Geometry check sheet. Reference: drawing and pictorial views, mm from the part's lowest x, y, z. Round coordinates to 2 decimals unless told otherwise and drop trailing zeros. Order: outer loops, then holes, each group sorted by start corner. A loop starts at its lowest first (then second) coordinate and runs counter-clockwise, first axis right, second up.
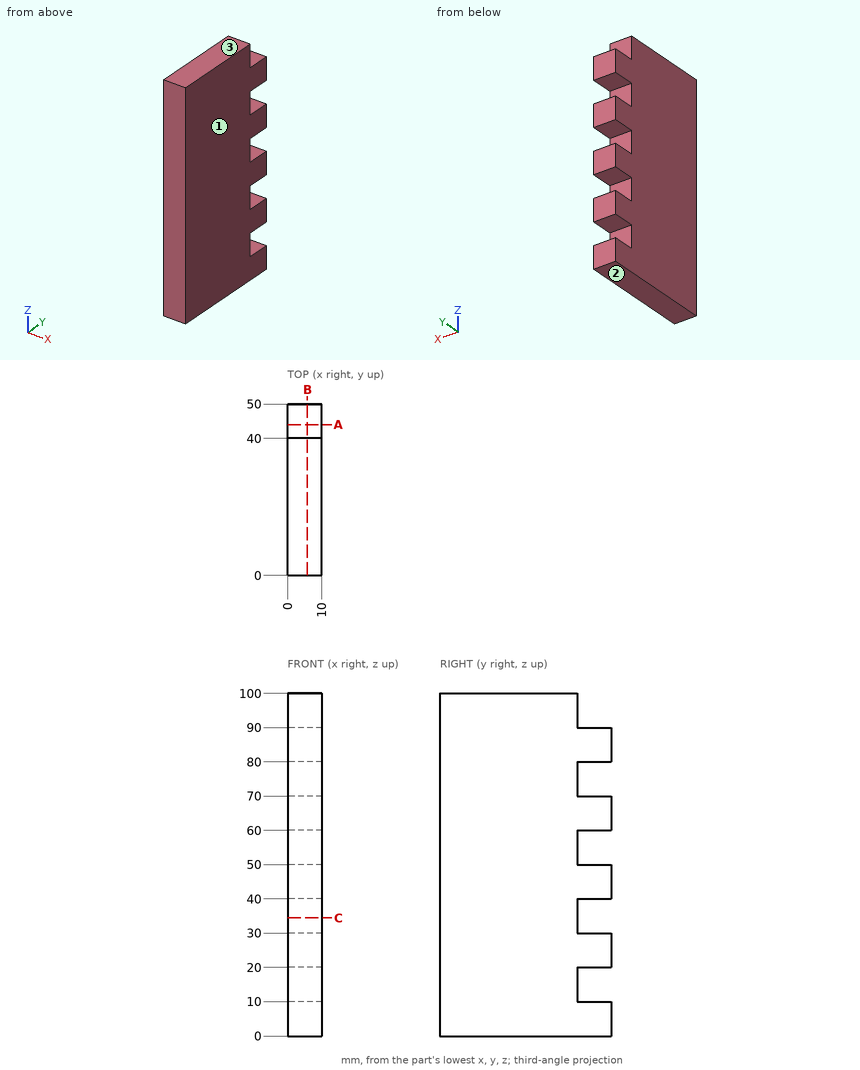
1) Go/stop test with flat-tipped pins: pin 1 Ø4 at (x, z) = (1, 34) entering from +Y; pin 2 Ø2 at (x, y) = (5.5, 32) entering from -Z; pin 3 Ø3 at (x, y) = (6.5, 43.5) entering from +Z. Record where each tip stops, or that it passes through.
2) Draft check along Z on the marked faces 1, 2 and 3. Enter one of: released by +Z, released by -Z, zero draft, split by the parting line, or undercut.
3) Sectioned sample at B-B on x = 5.75. Record the cut outline in (y, z).
4) Sectioned sample at C-C on z = 34.5. Record the cut outline in (x, y), then the cut area to 3 significant figures.
5) Scan lines: probe 1 along Z at (x, y) = (3, 41); probe 2 along Y at (x, z) = (8.5, 93). Record each from-to range of solid material in increasing order.
6) Sectioned sample at A-A on y = 44. Record the cut outline in (x, z).
Returned:
1. pin 1: stops at y = 40
1. pin 2: stops at z = 0
1. pin 3: stops at z = 90
2. face 1: zero draft
2. face 2: released by -Z
2. face 3: released by +Z
3. outline: (0, 0) - (50, 0) - (50, 10) - (40, 10) - (40, 20) - (50, 20) - (50, 30) - (40, 30) - (40, 40) - (50, 40) - (50, 50) - (40, 50) - (40, 60) - (50, 60) - (50, 70) - (40, 70) - (40, 80) - (50, 80) - (50, 90) - (40, 90) - (40, 100) - (0, 100) - close
4. outline: (0, 0) - (10, 0) - (10, 40) - (0, 40) - close
4. area: 400 mm2
5. probe 1: z = 0 to 10, 20 to 30, 40 to 50, 60 to 70, 80 to 90
5. probe 2: y = 0 to 40
6. outline: (0, 0) - (10, 0) - (10, 10) - (0, 10) - close; (0, 20) - (10, 20) - (10, 30) - (0, 30) - close; (0, 40) - (10, 40) - (10, 50) - (0, 50) - close; (0, 60) - (10, 60) - (10, 70) - (0, 70) - close; (0, 80) - (10, 80) - (10, 90) - (0, 90) - close
